Source: three-view drawing plus pictorial views. Frame: mm from the lowest corner of the part. Coordinates: 2 decimals unless noted, no trailing zeros. Order: outer loops, then holes, each group sorted by start corner. A loop starts at its lowest first (then second) coordinate and runs counter-clockwise, first axis right, second up. Notation, with made-up numbers: (78, 89) - (86, 89) arc R14 cw to (86, 103) - close; hole circle Ø9 at (39, 88). An arc over 180 degrees is marked (long way). One line per question, with ' | ' between items.
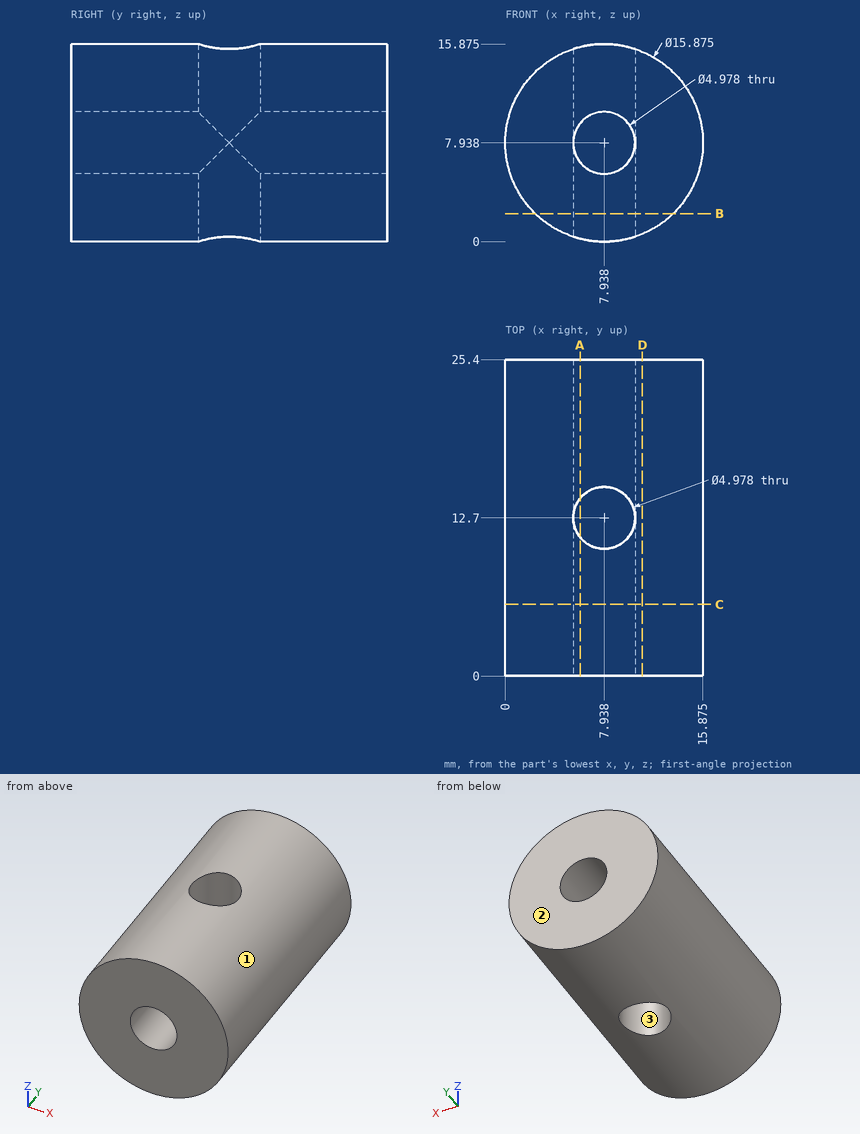
(1) Cut plane C-C (y = 5.75). Return the cut outline in (x, z) (1 decimal).
Taken from the geometry:
outline: circle Ø15.9 at (7.9, 7.9); hole circle Ø5 at (7.9, 7.9)
(2) Cut plane D-D (x = 11). Return the cut outline in (y, z) (1 decimal).
Taken from the geometry:
outline: (0, 0.6) - (25.4, 0.6) - (25.4, 15.3) - (0, 15.3) - close
(3) Pin query (flat end, axial travel): P1, Ø4, axis at x = 13.5, y = 16.5, coming from the +Z side; P2, Ø5, axis at y = 13.5, z = 12, coming from the -X side (1 decimal); P3, Ø1, axis at x = 3.5, y = 7, coming from the -Z side (1 decimal). Return the tip coordinate at first contact, or that it passes through.
Taken from the geometry:
P1: stops at z = 15.03 | P2: stops at x = 0.2 | P3: stops at z = 1
(4) Cut plane B-B (z = 2.25). Return the cut outline in (x, y) (1 decimal).
Taken from the geometry:
outline: (2.4, 0) - (13.5, 0) - (13.5, 25.4) - (2.4, 25.4) - close; hole circle Ø5 at (7.9, 12.7)
(5) Material intervals for L1, parallel to Y at x = 8, z = 12.5; L2, parallel to X at y = 1, z = 9.75 (1 decimal); L3, parallel to Z at x = 7.25, y = 18 (1 decimal), sorted ascending. Write a range as from..to.
Taken from the geometry:
L1: y = 0..10.21, 15.19..25.4 | L2: x = 0.2..6.2, 9.6..15.7 | L3: z = 0..5.5, 10.3..15.8
(6) Pull-direction query (X, two-part tool) for the marked faces 1, 2 and 3; classes: pulls with the +X half, pulls with the -X half, needs draft (parallel to the pull), parting line crosses it, or undercut.
Taken from the geometry:
face 1: parting line crosses it | face 2: needs draft | face 3: undercut
(7) Cut plane A-A (x = 6). Return the cut outline in (y, z) (1 decimal), and give its area (3 significant figures).
Taken from the geometry:
outline: (0, 0.2) - (11.1, 0.2) - (11.1, 6.4) - (0, 6.4) - close; (0, 9.5) - (11.1, 9.5) - (11.1, 15.6) - (0, 15.6) - close; (14.3, 0.2) - (25.4, 0.2) - (25.4, 6.4) - (14.3, 6.4) - close; (14.3, 9.5) - (25.4, 9.5) - (25.4, 15.6) - (14.3, 15.6) - close | area: 273 mm²
